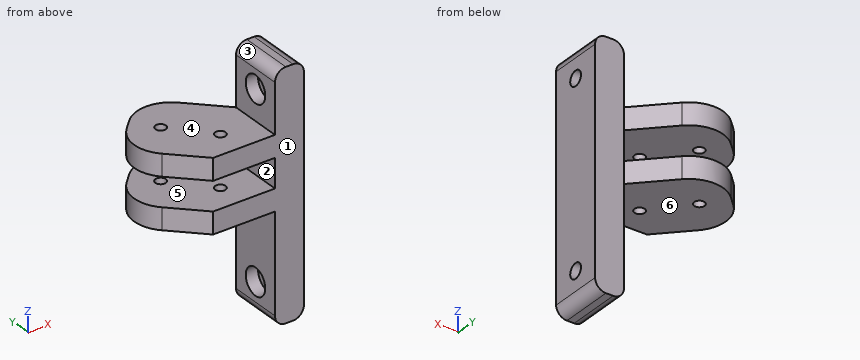
Autodesk Inventor part; units mm, degrees
ref_plane "Work Plane1" through (0, -6.5, 0) normal (0, 1, 0) x (-1, 0, 0)
ref_plane "Work Plane2" through (-7, -6.5, 8.75) normal (0, 0, -1) x (-1, 0, 0)
ref_plane "Work Plane3" through (-2.625, -6.5, 2.825) normal (0, 0, -1) x (-1, 0, 0)
ref_plane "Work Plane1" through (0, -6.5, 0) normal (0, 1, 0) x (-1, 0, 0)
sketch "Sketch1" plane through (0, -6.5, 0) normal (0, 1, 0) x (-1, 0, 0)
  line L0 (0, 0) -> (0, 29.475)
  arc A0 (2.625, 32.1) -> (0, 29.475) centre (2.625, 29.475) ccw
  line L1 (7, 29.475) -> (7, 17.5)
  line L2 (22, 12.25) -> (7, 12.25)
  line L3 (2.625, 32.1) -> (4.375, 32.1)
  line L4 (7, 12.25) -> (7, 5.25)
  arc A1 (7, 29.475) -> (4.375, 32.1) centre (4.375, 29.475) ccw
  line L5 (7, 17.5) -> (22, 17.5)
  line L6 (22, 0) -> (0, 0)
  line L7 (7, 5.25) -> (22, 5.25)
  line L8 (0, 0) -> (7, 0)
  line L9 (7, 0) -> (7, -23.825)
  line L10 (4.375, -26.45) -> (2.625, -26.45)
  line L11 (0, -23.825) -> (0, 0)
  arc A2 (0, -23.825) -> (2.625, -26.45) centre (2.625, -23.825) ccw
  arc A3 (4.375, -26.45) -> (7, -23.825) centre (4.375, -23.825) ccw
  line L12 (22, 17.5) -> (22, 12.25)
  line L13 (22, 5.25) -> (22, 0)
  point P0 (0, 0)
  point P1 (7, 0)
  dimension "d35" = 7
  dimension "d36" = 7
  dimension "d38" = 5.25
  dimension "d39" = 14.6
  dimension "d48" = 2.625
  dimension "d49" = 2.625
  dimension "d50" = 23.825
  dimension "d53" = 15
extrude "Extrusion2" add sketch "Sketch1" along normal blind 13
hole "Hole3" at (-15.5, 0, 12.25) direction (0, 0, 1) diameter 2.529 depth 5.25
sketch "Sketch3" plane through (-7, -6.5, 12.25) normal (0, 0, -1) x (-1, 0, 0)
  line L0 (0, 0) -> (0, 13)
  line L1 (0, 13) -> (15, 13)
  point P0 (8.5, 6.5)
  point P1 (12.375, 13)
  dimension "d51" = 8.5
  dimension "d52" = 6.5
hole "Hole1" at (-15.5, 0, 0) direction (0, 0, 1) diameter 2.529 depth 5.25
sketch "Sketch6" plane through (-19.375, -6.5, 17.5) normal (0, 0, 1) x (1, 0, 0)
  circle A0 centre (-4.0623, 15.5) radius 4.5
  circle A1 centre (3.875, 6.5) radius 4.5
  circle A2 centre (3.875, 6.5) radius 1.2645
  line L0 (-2.625, 0) -> (12.375, 0)
  line L1 (12.375, 0) -> (12.375, 13)
  line L2 (-2.625, 13) -> (12.375, 13)
  circle A3 centre (3.875, 6.5) radius 1.2645
  circle A4 centre (-4.0623, 15.5) radius 6.5
  circle A5 centre (3.875, 6.5) radius 6.5
  line L3 (3.875, 11) -> (-4.0623, 11)
  line L4 (0, 0) -> (0, 0)
  line L5 (0, 0) -> (0, 13)
  line L6 (0, 13) -> (0, 13)
  line L7 (0, 0) -> (0, 13)
  line L8 (-2.625, 0) -> (-2.625, 13.3311)
  line L9 (-2.625, 0) -> (-15.6685, 13.1351)
  line L10 (-15.6685, 13.1351) -> (-1.6162, 27.0894)
  line L11 (12.375, 0) -> (12.375, 13)
  line L12 (-1.6162, 27.0894) -> (12.375, 13)
  line L13 (2.9639, 22.4772) -> (-11.0884, 8.5228)
  circle A6 centre (-4.0623, 15.5) radius 1.2645
  line L14 (-2.625, 0) -> (-2.625, 13)
  point P0 (19.375, 6.5)
  point P1 (-2.625, 11)
  point P2 (-0.8154, 11)
  point P3 (-2.625, 1.1851)
  point P4 (3.875, 13)
  point P5 (3.875, 0)
  point P6 (-2.625, 11)
  point P7 (-2.625, 6.5)
  dimension "d26" = 9
  dimension "d27" = 9
  dimension "d28" = 2
  dimension "d29" = 2
  dimension "d30" = 1
extrude "Extrusion4" add sketch "Sketch6" against normal up to surface (5.25 mm away) contours A0 L2 L8 L13 A6 | A0 L13 A4 L2 | L13 A6 A0 | A0 L13 A4 | L2 L5 A5 L3 L8 A0 | A0 L8 L2 | A0 L3 L8 A4 L13 | L13 L12 L2 A4 | A4 L10 L12 L13 | L8 L3 A0 | L2 A4 A5 L5 | L13 L9 L10 A4 | A4 L8 L9 L13 | L3 A5 A4 L8 | L2 A5 A4 | L5 L3 A5 | A5 A4 L3 L5 | A4 A5 L8 | L1 L0 A5 L2 | L3 L5 A4 A5 | A5 L5 A1 L3 A4 | L3 A4 L5 | A4 L5 A1 A5 | A5 L5 L0 L8 | L3 A1 L5 A4 | A5 L0 L5 | A1 L5 | L5 A1
ref_plane "Work Plane2" through (-7, -6.5, 8.75) normal (0, 0, -1) x (-1, 0, 0)
mirror "Mirror1" about plane through (-7, -6.5, 8.75) normal (0, 0, -1) of "Extrusion4"
fillet "Fillet1" radius 8.35 4 edges at (-35.0435, 6.6351, 14.875) (-20.9912, 20.5894, 14.875) (-20.9912, 20.5894, 2.625) (-35.0435, 6.6351, 2.625)
sketch "Sketch8" plane through (-7, -6.5, 5.25) normal (-1, 0, 0) x (0, 0, 1)
  line L0 (0, 0) -> (7, 0)
  line L1 (7, 0) -> (7, 13)
  line L2 (0, 13) -> (7, 13)
  line L3 (0, 0) -> (0, 13)
  line L4 (12.25, 0) -> (24.225, 0)
  line L5 (24.225, 0) -> (24.225, 13)
  line L6 (12.25, 13) -> (24.225, 13)
  line L7 (12.25, 0) -> (12.25, 13)
  line L8 (24.225, 0) -> (26.85, 0)
  line L9 (26.85, 0) -> (26.85, 13)
  line L10 (24.225, 13) -> (26.85, 13)
  line L11 (24.225, 0) -> (24.225, 13)
  line L12 (26.85, 0) -> (26.85, 13) construction
  line L13 (26.85, 13) -> (12.25, 0) construction
  point P0 (-5.25, 6.5)
  point P1 (19.55, 6.5)
  point P2 (19.55, 6.5)
hole "Hole5" at (-7, 0, 24.8) direction (1, 0, 0) diameter 3.6 end through all counterbore diameter 6.5 counterbore depth 3
ref_plane "Work Plane3" through (-2.625, -6.5, 2.825) normal (0, 0, -1) x (-1, 0, 0)
mirror "Mirror2" about plane through (-2.625, -6.5, 2.825) normal (0, 0, -1) of "Hole5"
sketch "Sketch5" plane through (0, -6.5, 0) normal (0, 0, -1) x (-1, 0, 0)
  circle A0 centre (15.5, 6.5) radius 1.2645
ref_plane "Work Plane4" through (-2.625, -6.5, 2.825) normal (0, 0, -1) x (-1, 0, 0)
properties part number "Idle belt holder"
Could you check a few things on this model? Use its own coordinates, in mm. Face numbers are marked on the shaded views. A direction names the side the tool comes from. Coordinates: 2 decimals unless noted, no trailing zeros. Loops run counter-clockwise (first coordinate to the right, second up) from the corner with the lowest first, then second, coordinate; pieces in that order, holes last.
1. Imagine slicing it at B-B (x = -23). Please give me the cut outline in (y, z).
2. For P1, Ø5, axis at x = -26.5, y = 9, coming from the -Z side; P2, Ø1.5, axis at y = 4, z = -8.5, coming from the -X side; P3, Ø2, axis at y = -1, z = 25, coming from the -X side, each with a flat end and sliding along its axis, tell me the tip position at first contact or that it passes through.
3. I need wall thicknesses on L1, parallel to Z at x = -17, y = 12.75; L2, parallel to X at y = 2.25, z = 23; L3, parallel to Y at x = -6.5, z = 5. Which ranges of each line are inside material? Lowest first, please.
4. For the marked faces 4, 5 and 6, which set-ups out of +Z, -Z, +X, -X, +Y, -Y let a thin tool reach every point of the face, with its end or its side?
5. We'd pull the mould along Z, two halves only. Please class the marked faces 1, 2 and 3: released by +Z, released by -Z, zero draft, split by the parting line, or undercut.
6. Imagine slicing it at C-C (y = 9). Please give me the cut outline in (x, z), and give its area (3 significant figures).
7. Imagine slicing it at D-D (x = -27.5). Please give me the cut outline in (y, z), and give its area (3 significant figures).
8. Imagine slicing it at A-A (z = 24.8). Please give me the cut outline in (x, y), and give its area (3 significant figures).
Computed values:
1. outline: (-5.49, 0) - (7.81, 0) - (7.81, 5.25) - (-5.49, 5.25) - close; (-5.49, 12.25) - (7.81, 12.25) - (7.81, 17.5) - (-5.49, 17.5) - close; (10.19, 0) - (16.9, 0) - (16.9, 5.25) - (10.19, 5.25) - close; (10.19, 12.25) - (16.9, 12.25) - (16.9, 17.5) - (10.19, 17.5) - close
2. P1: stops at z = 0
2. P2: stops at x = -7
2. P3: stops at x = -4
3. L1: z = 0 to 5.25, 12.25 to 17.5
3. L2: x = -4 to 0
3. L3: y = -6.5 to 6.5
4. face 4: +Z, -X, +Y, -Y
4. face 5: -X, +Y, -Y
4. face 6: -Z, -X, +Y, -Y
5. face 1: zero draft
5. face 2: undercut
5. face 3: released by +Z
6. outline: (-31.23, 0) - (-24.7, 0) - (-24.7, 5.25) - (-31.23, 5.25) - close; (-31.23, 12.25) - (-24.7, 12.25) - (-24.7, 17.5) - (-31.23, 17.5) - close; (-22.17, 0) - (-9.48, 0) - (-9.48, 5.25) - (-22.17, 5.25) - close; (-22.17, 12.25) - (-9.48, 12.25) - (-9.48, 17.5) - (-22.17, 17.5) - close
6. area: 202 mm2
7. outline: (-0.96, 0) - (14.13, 0) - (14.13, 5.25) - (-0.96, 5.25) - close; (-0.96, 12.25) - (14.13, 12.25) - (14.13, 17.5) - (-0.96, 17.5) - close
7. area: 158 mm2
8. outline: (-7, -6.5) - (0, -6.5) - (0, -1.8) - (-4, -1.8) - (-4, -3.25) - (-7, -3.25) - close; (-7, 3.25) - (-4, 3.25) - (-4, 1.8) - (0, 1.8) - (0, 6.5) - (-7, 6.5) - close
8. area: 57.1 mm2
